Can you work these out from the model? Positions are in its coordinate system, mm. A direction names the side the tool comes from. Coordinates: 2 decimals unless noted, no trailing zeros. Write each loop counter-clockwise with the first axis right and the second up, starting at its lowest first coordinate (ties: lowest second). Pieces come first, ordered by that corner, then holes. Notation, with made-up numbers: (77, 82) - (86, 82) arc R8 ccw to (86, 91) - close; hole circle Ø9 at (27, 52). An arc over 180 degrees is marked (long way). One line per question, with ' | ' between items. Start each with the question number.
from build123d import *

# Parameters (mm, degrees)
SKETCH1_R           = 10
SKETCH1_R_2         = 7.5
BOSS_EXTRUDE1_DEPTH = 5
BOSS_EXTRUDE2_START = 1
SKETCH1_3_R         = 10
SKETCH1_3_R_2       = 7.5
SKETCH1_3_R_3       = 4.5
BOSS_EXTRUDE2_DEPTH = 1
SKETCH2_R           = 10
BOSS_EXTRUDE3_DEPTH = 6
BOSS_EXTRUDE7_REACH = 67.117
SKETCH3_W           = 15
SKETCH3_H           = 14
SKETCH4_R           = 2
CUT_EXTRUDE4_DEPTH  = 68.647985927
CUT_EXTRUDE5_START  = 3
SKETCH4_3_R         = 2
CUT_EXTRUDE5_DEPTH  = 65.647985927
BOSS_EXTRUDE8_REACH = 69.648


with BuildPart() as part:
    # Sketch1 → Boss-Extrude1 (new body)
    with BuildSketch(Plane.XY):
        Circle(SKETCH1_R)
        Circle(SKETCH1_R_2, mode=Mode.SUBTRACT)
    extrude(amount=-BOSS_EXTRUDE1_DEPTH)

    # Sketch1<3> → Boss-Extrude2 (add)
    # profile 1 of 2: a face of its own
    with BuildSketch(Plane.XY.offset(BOSS_EXTRUDE2_START)):
        Circle(SKETCH1_3_R)
        Circle(SKETCH1_3_R_2, mode=Mode.SUBTRACT)
    # profile 2 of 2: a face of its own
    with BuildSketch(Plane.XY.offset(BOSS_EXTRUDE2_START)):
        Circle(SKETCH1_3_R_2)
        Circle(SKETCH1_3_R_3, mode=Mode.SUBTRACT)
    extrude(amount=-BOSS_EXTRUDE2_DEPTH)

    # Sketch2 → Boss-Extrude3 (add)
    with BuildSketch(Plane.XY.offset(1)):
        Polygon((55, 17.5), (55, 22.5), (40, 22.5), (40, 36.2), (-12, 11.952001776), (-12, -12), (12, -12), (12, -2.551229301), align=None)
        Circle(SKETCH2_R, mode=Mode.SUBTRACT)
    extrude(amount=-BOSS_EXTRUDE3_DEPTH)

    # Boss-Extrude7: up to this plane
    boss_extrude7_end = Plane(origin=(3.120451856, -6.691830601, -87.536295046), z_dir=(-0.422618261740692, 0.9063077870366535, 0))
    # Sketch3 → Boss-Extrude7 (add, up to the surface)
    with BuildSketch(Plane.XZ.offset(-22.5), mode=Mode.PRIVATE) as boss_extrude7_sk1:
        Polygon((40, -5), (40, -19), (10.620255189, -5), align=None)
    boss_extrude7_tool1 = split(extrude(boss_extrude7_sk1.sketch, amount=BOSS_EXTRUDE7_REACH, mode=Mode.PRIVATE), bisect_by=boss_extrude7_end, keep=Keep.BOTH, mode=Mode.PRIVATE)
    add(boss_extrude7_tool1.solids().sort_by_distance((30.206752, 22.5, -9.666667))[0])
    # Sketch3 → Boss-Extrude7 (add, up to the surface)
    with BuildSketch(Plane.XZ.offset(-22.5), mode=Mode.PRIVATE) as boss_extrude7_sk2:
        with Locations((47.5, -12)):
            Rectangle(SKETCH3_W, SKETCH3_H)
    boss_extrude7_tool2 = split(extrude(boss_extrude7_sk2.sketch, amount=BOSS_EXTRUDE7_REACH, mode=Mode.PRIVATE), bisect_by=boss_extrude7_end, keep=Keep.BOTH, mode=Mode.PRIVATE)
    add(boss_extrude7_tool2.solids().sort_by_distance((47.5, 22.5, -12))[0])

    # Sketch4 → Cut-Extrude4 (cut, through all)
    with BuildSketch(Plane.XZ.offset(-22.5)):
        with Locations((47.5, -14)):
            Circle(SKETCH4_R)
        with Locations((47.5, -4)):
            Circle(SKETCH4_R)
    extrude(amount=CUT_EXTRUDE4_DEPTH, mode=Mode.SUBTRACT)

    # Sketch4<3> → Cut-Extrude5 (cut, through all)
    # profile 1 of 2: a face of its own
    with BuildSketch(Plane.XZ.offset(-22.5).offset(CUT_EXTRUDE5_START)):
        Polygon((47.5, -8.041451884), (44, -6.020725942), (44, -1.979274058), (47.5, 0.041451884), (51, -1.979274058), (51, -6.020725942), align=None)
        with Locations(Location((47.5, -4, 0), (0, 0, 270))):
            Circle(SKETCH4_3_R, mode=Mode.SUBTRACT)
    # profile 2 of 2: a face of its own
    with BuildSketch(Plane.XZ.offset(-22.5).offset(CUT_EXTRUDE5_START)):
        Polygon((51, -16.020725942), (51, -11.979274058), (47.5, -9.958548116), (44, -11.979274058), (44, -16.020725942), (47.5, -18.041451884), align=None)
        with Locations(Location((47.5, -14, 0), (0, 0, 270))):
            Circle(SKETCH4_3_R, mode=Mode.SUBTRACT)
    extrude(amount=CUT_EXTRUDE5_DEPTH, mode=Mode.SUBTRACT)

    # Boss-Extrude8: up to this face of the body (flat: up to its plane)
    boss_extrude8_end = Plane(part.part.faces().sort_by_distance((14, 24.076000888, -2))[0])
    # Sketch3<4> → Boss-Extrude8 (add, up to the picked face)
    with BuildSketch(Plane.XZ.offset(-22.5), mode=Mode.PRIVATE) as boss_extrude8_sk1:
        Polygon((40, -5), (40, -19), (10.620255189, -5), align=None)
    boss_extrude8_tool1 = split(extrude(boss_extrude8_sk1.sketch, amount=-BOSS_EXTRUDE8_REACH, mode=Mode.PRIVATE), bisect_by=boss_extrude8_end, keep=Keep.BOTH, mode=Mode.PRIVATE)
    add(boss_extrude8_tool1.solids().sort_by(Axis((30.206752, 22.5, -9.666667), (0, 1, 0)))[0])


solid = part.part
(1) If we section it at C-C on z = -13.25: List the corners of the cut face in (x, y) for me, plus the area to 3 significant figures.
(2) I'm going to push flat-ended pins straight in: pin 1 (1.5 mm diameter, centred on x = 14.5, y = 0, fed in from -Z); pin 2 (4.5 mm diameter, centred on y = 17, z = -5, fed in from -X); pin 3 (5.5 mm diameter, centred on x = 0, y = 0, fed in from -Z); pin 4 (4.5 mm diameter, centred on y = 18.5, z = -14.5, fed in from -X). Where does each tip first touch, or does it pass through?
(3) If we section it at B-B on y = 0: List the corners of the cut face in (x, z) for me, plus the area to 3 significant figures.
(4) Which directions (+Z, -Z, +X, -X, +Y, -Y) give clear straight access to the entire face, cutting with the end or side of a thin tool? Please do faces 4 (the face through (51, 18, -14)), 5 (the face through (55, 20, -9)), 6 (the face through (40, 29, -9)).
(5) If we section it at A-A on z = -4: List the corners of the cut face in (x, y) for me.
(6) If we mould it in two halves opening along X, with no side actions, what happens to faces 1 (the face through (47, 22.5, -9)), 2 (the face through (12, -7, -2)), 3 (the face through (-7.493, 0.33, -2.465))? For each: +X half, -X half, draft (parallel to the pull), parting line (faces both ways), or undercut.
(7) If I drill on probe 1 along Z at (x, y) = (47.5, 21.2); probe 2 along Z at (x, y) = (47, 20); probe 3 along Z at (x, y) = (-9, -7.5), over which ranges is the centre line in solid material (lowest first)?
(8) If we section it at D-D on x = 0: List the corners of the cut face in (y, z) for me, plus the area to 3 significant figures.
Values:
1) outline: (27.93, 4.88) - (44, 12.37) - (44, 19.5) - (45.65, 19.5) - (45.65, 22.5) - (40, 22.5) - (40, 36.2) - (27.93, 30.57) - close; (49.35, 19.5) - (51, 19.5) - (51, 15.63) - (55, 17.5) - (55, 22.5) - (49.35, 22.5) - close | area: 388 mm2
2) pin 1: z = -7.21 | pin 2: x = -6 | pin 3: through | pin 4: x = 25.83
3) outline: (-12, -5) - (-7.5, -5) - (-7.5, 0) - (-4.5, 0) - (-4.5, 1) - (-12, 1) - close; (4.5, 0) - (7.5, 0) - (7.5, -5) - (10.62, -5) - (17.47, -8.26) - (17.47, 1) - (4.5, 1) - close | area: 104 mm2
4) face 4: -Y | face 5: +Z, -Z, +X, +Y, -Y | face 6: +Z, -Z, +X, +Y
5) outline: (-12, -12) - (12, -12) - (12, -2.55) - (44, 12.37) - (44, 19.5) - (45.5, 19.5) - (45.5, 22.5) - (40, 22.5) - (40, 36.2) - (-12, 11.95) - close; (49.5, 19.5) - (51, 19.5) - (51, 15.63) - (55, 17.5) - (55, 22.5) - (49.5, 22.5) - close; hole circle Ø15 at (0, 0)
6) face 1: draft | face 2: +X half | face 3: undercut
7) probe 1: -19 to -16, -12 to -6, -2 to 1 | probe 2: -19 to -15.94, -12.06 to -5.94, -2.06 to 1 | probe 3: -5 to 1
8) outline: (-12, -5) - (-7.5, -5) - (-7.5, 0) - (-4.5, 0) - (-4.5, 1) - (-12, 1) - close; (4.5, 0) - (7.5, 0) - (7.5, -5) - (17.55, -5) - (17.55, 1) - (4.5, 1) - close | area: 93.3 mm2
